from build123d import *

# Parameters (mm, degrees)
SKETCH1_R           = 15.9131
BASEPULLEY_DEPTH    = 10.414
GROOVE_DEPTH        = 5.207
GROOVES_COUNT       = 20
GROOVES_ANGLE       = 342
SKETCH4_W           = 0.254
SKETCH4_H           = 11.43
BORSKE_R            = 3.175
BORE_DEPTH          = 27.855010035
SKETCH7_R           = 16.713739002
SKETCH7_R_2         = 3.214245881
BOSS_EXTRUDE1_DEPTH = 0.254


with BuildPart() as part:
    # Sketch1 → BasePulley (new body)
    with BuildSketch(Plane.XY):
        Circle(SKETCH1_R)
    extrude(amount=-BASEPULLEY_DEPTH)

    # Sketch2 → Flange (revolve)
    with BuildSketch(Plane(origin=(0, 0, 0), x_dir=(0, 0, -1), z_dir=(1, 0, 0)), mode=Mode.PRIVATE) as flange_sk:
        Polygon((10.414, 15.9131), (10.724622372, 16.9291), (11.429036456, 16.713739002), (11.1506, 15.803014392), (11.1506, 0), (-0.7366, 0), (-0.7366, 15.803014392), (-1.015036456, 16.713739002), (-0.310622372, 16.9291), (0, 15.9131), align=None)
    revolve(flange_sk.sketch.rotate(Axis((0, 0, 0), (0, 0, -1)), 90), axis=Axis((0, 0, 0), (0, 0, -1)))

    # Sketch3 → Groove (cut, symmetric)
    with BuildSketch(Plane.XY.offset(-5.207)):
        with BuildLine():
            Line((-1.2827, 15.9131), (-1.2827, 41.3131))
            Line((-1.2827, 41.3131), (1.2827, 41.3131))
            Line((1.2827, 41.3131), (1.2827, 15.9131))
            Line((1.2827, 15.9131), (0.659450384, 14.8336))
            ThreePointArc((0.659450384, 14.8336), (0.519994706, 14.694144321), (0.329494706, 14.6431))
            Line((0.329494706, 14.6431), (-0.55367873, 14.6431))
            ThreePointArc((-0.55367873, 14.6431), (-0.772211353, 14.712003071), (-0.911701619, 14.893790325))
            Line((-0.911701619, 14.893790325), (-1.2827, 15.9131))
        make_face()
    groove = extrude(amount=GROOVE_DEPTH, both=True, mode=Mode.SUBTRACT)

    # Grooves: Groove ×20 about axis
    grooves_axis = Axis((0, 0, -10.414), (0, 0, 1))
    for i in range(1, GROOVES_COUNT):
        add(groove.rotate(grooves_axis, i * GROOVES_ANGLE / (GROOVES_COUNT - 1)), mode=Mode.SUBTRACT)

    # Sketch4 → BaseHub (revolve)
    with BuildSketch(Plane(origin=(0, 0, 0), x_dir=(0, 0, -1), z_dir=(1, 0, 0)), mode=Mode.PRIVATE) as basehub_sk:
        with Locations((-0.127, 5.715)):
            Rectangle(SKETCH4_W, SKETCH4_H)
    revolve(basehub_sk.sketch.rotate(Axis((0, 0, 0), (0, 0, -1)), 274.520210968), axis=Axis((0, 0, 0), (0, 0, -1)))

    # BorSke → Bore (cut, through all)
    with BuildSketch(Plane.XY.offset(0.7366)):
        Circle(BORSKE_R)
    extrude(amount=-BORE_DEPTH, mode=Mode.SUBTRACT)

    # Sketch7 → Boss-Extrude1 (add)
    with BuildSketch(Plane(origin=(0, 0, -11.1506), x_dir=(-1, 0, 0), z_dir=(0, 0, -1))):
        Circle(SKETCH7_R)
        Circle(SKETCH7_R_2, mode=Mode.SUBTRACT)
    extrude(amount=BOSS_EXTRUDE1_DEPTH)


solid = part.part
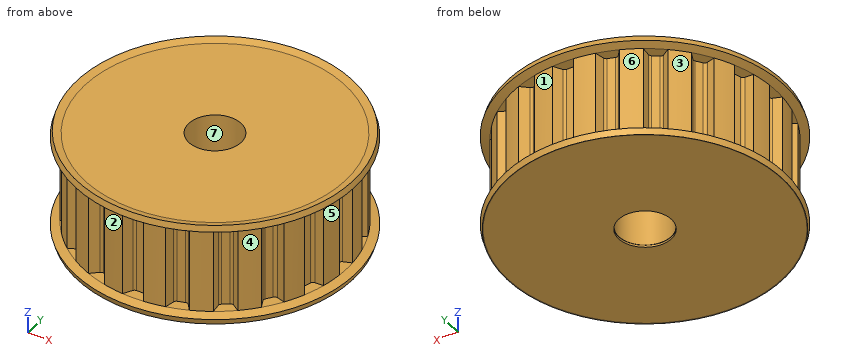
Work out the finished part from the listing and answer in its coordinate system (mm). Face numbers are marked on the shaded views. A direction names the side the tool comes from. Round coordinates to 2 decimals unless told otherwise and drop trailing zeros. Use a Markdown table: item, result.
1) Which of the six approach directions +Z, -Z, +X, -X, +Y, -Y give full straight-line access (tool end or side, diameter ignored) to the marked faces 1, 2, 3 and 4?
Taken from the geometry:
| item | result |
|---|---|
| face 1 | +X, +Y |
| face 2 | -X, -Y |
| face 3 | -X, +Y |
| face 4 | +X, -Y |
2) Consider line 1 (Y direction, x = 0, z = -7) (3 decimals); line 2 (Z direction, x = 7, y = 0.5); line 3 (Y direction, x = 0, z = -11.3). Determine where each line is inside the solid, lowest interval first. Write a range as [from, to].
Taken from the geometry:
| item | result |
|---|---|
| line 1 | y = [-14.643, -3.175], [3.175, 14.643] |
| line 2 | z = [-11.4, 0.74] |
| line 3 | y = [-16.75, -3.21], [3.21, 16.75] |
3) Flat-ended cylindrical pins translate along their axes: pin 1 (1.4 mm diameter, centred on x = 15.5, y = -0.5, fed in from -Z); pin 2 (1.1 mm diameter, centred on x = 9, y = -12, fed in from +Z); pin 3 (1.5 mm diameter, centred on x = -6.5, z = -2.5, fed in from +Y). Find the tip coordinate at first contact, or state that the pin passes through.
Taken from the geometry:
| item | result |
|---|---|
| pin 1 | stops at z = -11.4 |
| pin 2 | stops at z = 0.74 |
| pin 3 | stops at y = 14.7 |
4) Determine the mould class of the marked faces 5, 6 and 7 for opening direction X: pulls with the +X half, pulls with the -X half, needs draft (parallel to the pull), parting line crosses it, or undercut.
Taken from the geometry:
| item | result |
|---|---|
| face 5 | pulls with the +X half |
| face 6 | pulls with the -X half |
| face 7 | undercut |
